The drawing under review shows one solid part. Ordinate dimensions are in mm from its lowest x, y, z. A direction names the side the tool comes from. Coordinates: 2 decimals unless noted, no trailing zeros. Write each loop counter-clockwise with the first axis right and the second up, starting at its lowest first coordinate (ties: lowest second). Pieces come first, ordered by that corner, then holes. Notation, with made-up numbers: (37.5, 0) - (43.5, 0) arc R24 ccw to (43.5, 20) - close; hole circle Ø1 at (3.25, -13.5). An arc over 180 degrees is marked (long way). Answer as CSV lines item,"result". Start each with the question number.
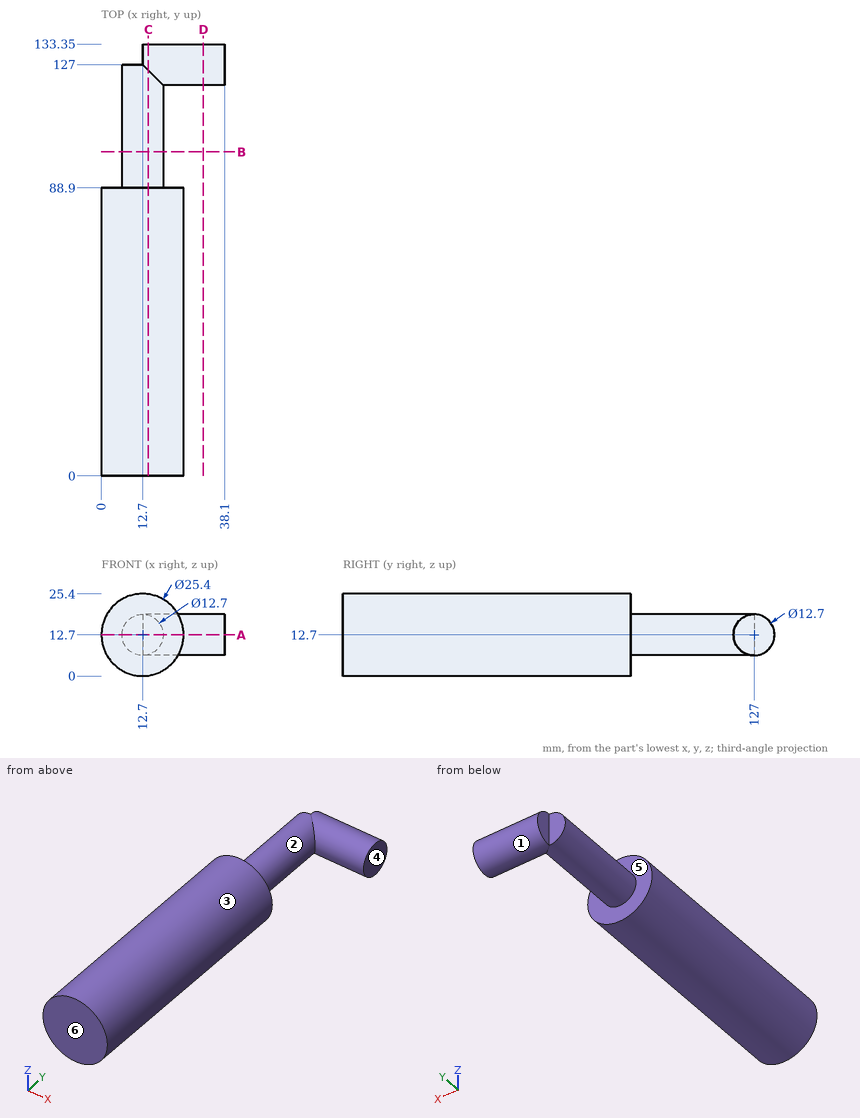
(1) Add section B-B on y = 100. Give the boundary of the cut face in (x, z).
(2) Add section A-A on z = 12.7. Give the boundary of the cut face in (x, y).
(3) The part is to be moulded in two halves that separate along Y. For the marked faces 4, 5 and 6, say which applies: released by +Y, released by -Y, zero draft, split by the parting line, or undercut.
(4) For the marked faces 1, 2 and 3, list the 3-axis set-ups (+Z, -Z, +X, -X, +Y, -Y) from which the entire face can be reached by the end or side of a thin tool; tool diameter is ignored.
(5) Add section C-C on x = 14.5. Give the boundary of the cut face in (y, z), then the cut area to 3 significant figures.
(6) Add section D-D on x = 31.5. Give the boundary of the cut face in (y, z).
(7) For pin 1 (5 mm diameter, centred on y = 44.5, z = 7.5, fed in from -X); pin 2 (5 mm diameter, centred on x = 8, z = 13.5, fed in from +Y); pin 3 (12 mm diameter, centred on x = 23, y = 101, fed in from -Z), all flat-tipped, find the tip position at first contact; note any pin that passes through.
(8) Wall thickness on line 1 (Y direction, x = 5, z = 3.75); line 2 (Y direction, x = 20.5, z = 17.25); line 3 (Y direction, x = 11, z = 15.5): over which ranges is each line inside the solid? List them lowest first.
Reported:
1,outline,"circle Ø12.7 at (12.7, 12.7)"
2,outline,"(0, 0) - (25.4, 0) - (25.4, 88.9) - (19.05, 88.9) - (19.05, 120.65) - (38.1, 120.65) - (38.1, 133.35) - (12.7, 133.35) - (12.7, 127) - (6.35, 127) - (6.35, 88.9) - (0, 88.9) - close"
3,face 4,"zero draft"
3,face 5,"undercut"
3,face 6,"released by -Y"
4,face 1,"+X"
4,face 2,"none"
4,face 3,"-Y"
5,outline,"(0, 0.13) - (88.9, 0.13) - (88.9, 6.61) - (125.2, 6.61) arc R6.35 ccw (long way) to (125.2, 18.79) - (88.9, 18.79) - (88.9, 25.27) - (0, 25.27) - close"
5,area,"2,760 mm²"
6,outline,"circle Ø12.7 at (127, 12.7)"
7,pin 1,"x = 0.29"
7,pin 2,"y = 127"
7,pin 3,"z = 8.03"
8,line 1,"0 to 88.9"
8,line 2,"0 to 88.9, 122.57 to 131.43"
8,line 3,"0 to 127"
